from build123d import *

# Parameters (mm, degrees)
SKETCH1_R           = 35.75
SKETCH1_R_2         = 34.75
BOSS_EXTRUDE1_DEPTH = 9.5
SKETCH3_R           = 34.75
BOSS_EXTRUDE2_DEPTH = 2
SKETCH4_W           = 38.5
SKETCH4_H           = 45.5
SKETCH4_W_2         = 36.5
SKETCH4_H_2         = 43.5
BOSS_EXTRUDE3_DEPTH = 70
SKETCH2_R           = 36.8
SKETCH2_R_2         = 34.75
BOSS_EXTRUDE4_DEPTH = 2
SKETCH5_R           = 36.8
SKETCH5_R_2         = 35.8
BOSS_EXTRUDE5_DEPTH = 110
BOSS_EXTRUDE6_START = -60.5
BOSS_EXTRUDE6_DEPTH = 60.5
SKETCH7_R           = 9
CUT_EXTRUDE1_DEPTH  = 5
BOSS_EXTRUDE7_DEPTH = 50


with BuildPart() as part:
    # Sketch1 → Boss-Extrude1 (new body)
    with BuildSketch(Plane(origin=(0, 0, 0), x_dir=(1, 0, 0), z_dir=(0, 1, 0))):
        with Locations(Location((0, 0, 0), (0, 0, 270))):
            Circle(SKETCH1_R)
        with Locations(Location((0, 0, 0), (0, 0, 270))):
            Circle(SKETCH1_R_2, mode=Mode.SUBTRACT)
    extrude(amount=BOSS_EXTRUDE1_DEPTH)

    # Sketch3 → Boss-Extrude2 (add)
    with BuildSketch(Plane.XZ):
        with Locations(Location((0, 0, 0), (0, 0, 270))):
            Circle(SKETCH3_R)
    extrude(amount=-BOSS_EXTRUDE2_DEPTH)

    # Sketch4 → Boss-Extrude3 (add)
    with BuildSketch(Plane(origin=(0, 2, 0), x_dir=(1, 0, 0), z_dir=(0, 1, 0))):
        with Locations((-8.327164466, 0)):
            Rectangle(SKETCH4_W, SKETCH4_H)
        with Locations((-8.327164466, 0)):
            Rectangle(SKETCH4_W_2, SKETCH4_H_2, mode=Mode.SUBTRACT)
    extrude(amount=BOSS_EXTRUDE3_DEPTH)

    # Sketch2 → Boss-Extrude4 (add)
    with BuildSketch(Plane(origin=(0, 9.5, 0), x_dir=(1, 0, 0), z_dir=(0, 1, 0))):
        with Locations(Location((0, 0, 0), (0, 0, 270))):
            Circle(SKETCH2_R)
        Circle(SKETCH2_R_2, mode=Mode.SUBTRACT)
    extrude(amount=BOSS_EXTRUDE4_DEPTH)

    # Sketch5 → Boss-Extrude5 (add)
    with BuildSketch(Plane(origin=(0, 11.5, 0), x_dir=(1, 0, 0), z_dir=(0, 1, 0))):
        with Locations(Location((0, 0, 0), (0, 0, 270))):
            Circle(SKETCH5_R)
        with Locations(Location((0, 0, 0), (0, 0, 270))):
            Circle(SKETCH5_R_2, mode=Mode.SUBTRACT)
    extrude(amount=BOSS_EXTRUDE5_DEPTH)

    # Sketch6 → Boss-Extrude6 (add)
    with BuildSketch(Plane(origin=(0, 72, 0), x_dir=(1, 0, 0), z_dir=(0, 1, 0)).offset(BOSS_EXTRUDE6_START)):
        with BuildLine():
            Line((-26.267851073, 22.75), (-27.061555926, 23.437410072))
            ThreePointArc((-27.061555926, 23.437410072), (-27.748330258, 22.620127494), (-28.410431306, 21.782731532))
            Line((-28.410431306, 21.782731532), (-27.577164466, 21.143852534))
            Line((-27.577164466, 21.143852534), (-26.267851073, 22.75))
        make_face()
        with BuildLine():
            Line((-26.267851073, -22.75), (-27.061555926, -23.437410072))
            ThreePointArc((-27.061555926, -23.437410072), (-27.748330258, -22.620127494), (-28.410431306, -21.782731532))
            Line((-28.410431306, -21.782731532), (-27.577164466, -21.143852534))
            Line((-27.577164466, -21.143852534), (-26.267851073, -22.75))
        make_face()
    extrude(amount=BOSS_EXTRUDE6_DEPTH)

    # Sketch7 → Cut-Extrude1 (cut)
    with BuildSketch(Plane(origin=(36.8, 0, 0), x_dir=(0, 0, -1), z_dir=(1, 0, 0))):
        with Locations((0, 20)):
            Circle(SKETCH7_R)
    extrude(amount=-CUT_EXTRUDE1_DEPTH, mode=Mode.SUBTRACT)

    # Sketch8 → Boss-Extrude7 (add)
    with BuildSketch(Plane(origin=(0, 72, 0), x_dir=(1, 0, 0), z_dir=(0, 1, 0))):
        Polygon((10.276388924, 21.396446609), (19.780640943, 30.900698628), (18.782256531, 31.316527778), (9.569282143, 22.103553391), align=None)
        Polygon((9.569282143, -22.103553391), (10.276388924, -21.396446609), (19.780640943, -30.900698628), (18.782256531, -31.316527778), align=None)
    extrude(amount=-BOSS_EXTRUDE7_DEPTH)


solid = part.part
Verification items for the finished model (mm, model axes). A direction names the side the tool comes from. Coordinates: 2 decimals unless noted, no trailing zeros. Order: outer loops, then holes, each group sorted by start corner. A loop starts at its lowest first (then second) coordinate and runs counter-clockwise, first axis right, second up.
1. Sectioned sample at B-B, the plane y = 57. Record the cut outline in (x, z).
Results found:
outline: circle Ø73.6 at (0, 0); hole (-28.41, -21.78) - (-27.58, -21.14) - (-27.58, 21.14) - (-28.41, 21.78) arc R35.8 ccw to start; hole (-27.06, -23.44) arc R35.8 ccw to (18.26, -30.79) - (10.22, -22.75) - (-26.27, -22.75) - close; hole (-27.06, 23.44) - (-26.27, 22.75) - (10.22, 22.75) - (18.26, 30.79) arc R35.8 ccw to start; hole (-26.58, -21.75) - (9.92, -21.75) - (9.92, 21.75) - (-26.58, 21.75) - close; hole (10.92, -22.04) - (19.14, -30.26) arc R35.8 ccw to (19.14, 30.26) - (10.92, 22.04) - close
2. Sectioned sample at A-A, the plane z = 0. Record the cut outline in (x, y).
Results found:
outline: (-36.8, 9.5) - (-35.75, 9.5) - (-35.75, 0) - (35.75, 0) - (35.75, 9.5) - (36.8, 9.5) - (36.8, 11) - (34.75, 11) - (34.75, 2) - (10.92, 2) - (10.92, 72) - (9.92, 72) - (9.92, 2) - (-26.58, 2) - (-26.58, 72) - (-27.58, 72) - (-27.58, 2) - (-34.75, 2) - (-34.75, 11.5) - (-35.8, 11.5) - (-35.8, 121.5) - (-36.8, 121.5) - close; (35.8, 29) - (36.8, 29) - (36.8, 121.5) - (35.8, 121.5) - close
3. Scan lines: line 1 (Z direction, x = 0.5, y = 20.5); line 2 (X direction, y = 36, z = 0); line 3 (Z direction, x = 0, y = 6). Record each from-to range of solid material in increasing order.
Results found:
line 1: z = -36.8 to -35.8, -22.75 to -21.75, 21.75 to 22.75, 35.8 to 36.8
line 2: x = -36.8 to -35.8, -27.58 to -26.58, 9.92 to 10.92, 35.8 to 36.8
line 3: z = -35.75 to -34.75, -22.75 to -21.75, 21.75 to 22.75, 34.75 to 35.75
4. Sectioned sample at C-C, the plane x = 0. Record the cut outline in (y, z), and give its area (3 significant figures).
Results found:
outline: (0, -35.75) - (9.5, -35.75) - (9.5, -36.8) - (121.5, -36.8) - (121.5, -35.8) - (11.5, -35.8) - (11.5, -34.75) - (2, -34.75) - (2, -22.75) - (72, -22.75) - (72, -21.75) - (2, -21.75) - (2, 21.75) - (72, 21.75) - (72, 22.75) - (2, 22.75) - (2, 34.75) - (11.5, 34.75) - (11.5, 35.8) - (121.5, 35.8) - (121.5, 36.8) - (9.5, 36.8) - (9.5, 35.75) - (0, 35.75) - close
area: 526 mm2
5. Go/stop test with flat-tipped pins: pin 1 Ø2 at (y, z) = (100.5, 27) entering from -X; pin 2 Ø2 at (x, z) = (24, -25) entering from +Y; pin 3 Ø22 at (y, z) = (36.5, 5.5) entering from -X; pin 4 Ø12 at (x, z) = (-22.5, 24) entering from +Y. Record where each tip stops, or that it passes through.
Results found:
pin 1: stops at x = -26.04
pin 2: stops at y = 11.5
pin 3: stops at x = -36.8
pin 4: stops at y = 121.5
6. Set-up check for faces 1 (the face through (36, 9.5, -6)), 2 (the face through (-35.3, 121.5, 8)), 3 (the face through (-35, 11.5, -2)): record each of +Z, -Z, +X, -X, +Y, -Y from which the full face is reachable in a straight line by a thin tool's end or side.
Results found:
face 1: -Y
face 2: +Z, -Z, +X, -X, +Y
face 3: +Y
7. Sectioned sample at D-D, the plane y = 20. Record the cut outline in (x, z), and give its area (3 significant figures).
Results found:
outline: (-27.06, -23.44) - (-26.27, -22.75) - (10.92, -22.75) - (10.92, 22.75) - (-26.27, 22.75) - (-27.06, 23.44) arc R35.8 cw to (34.65, 9) - (35.68, 9) arc R36.8 ccw (long way) to (35.68, -9) - (34.65, -9) arc R35.8 cw to start; hole (-28.41, -21.78) - (-27.58, -21.14) - (-27.58, 21.14) - (-28.41, 21.78) arc R35.8 ccw to start; hole (-26.58, -21.75) - (9.92, -21.75) - (9.92, 21.75) - (-26.58, 21.75) - close
area: 376 mm2
